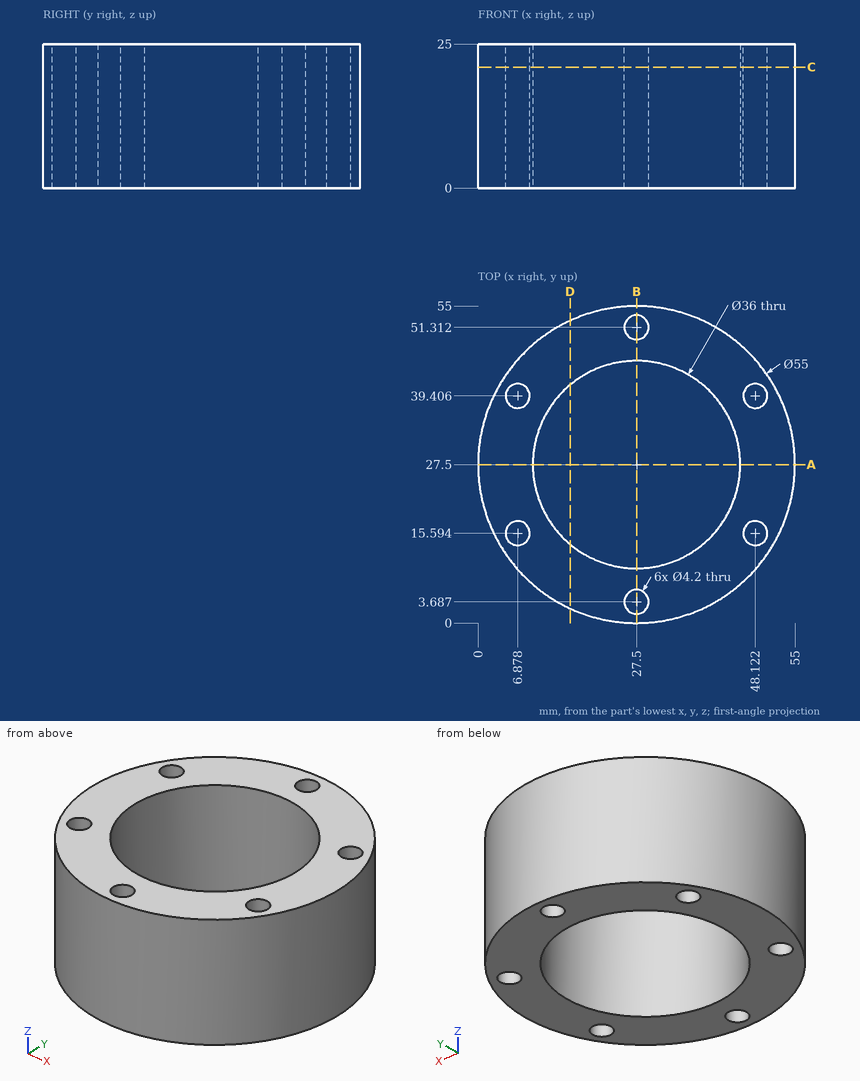
Geometry check sheet. Reference: drawing and pictorial views, mm from the part's lowest x, y, z. Give positions to 0.01 mm unless a question says otherwise; leave off trailing zeros. Write each loop counter-clockwise with the first axis right and the second up, starting at its lowest first coordinate (ties: lowest second). Pieces come first, ordered by that corner, then holes.
Item 1: Gauge pin test, flat ends, axial feed: pin 1 (4 mm diameter, centred on x = 48.12, y = 15.59, fed in from +Z); pin 2 (4 mm diameter, centred on x = 24, z = 15, fed in from -Y); pin 3 (8 mm diameter, centred on x = 6, y = 38, fed in from +Z); pin 4 (1.5 mm diameter, centred on x = 22.5, z = 14.5, fed in from +Y). Record the tip position at first contact, or that the pin passes through.
Item 2: Cross-section at A-A (y = 27.5). Enter the section's corners in (x, z), and give its area (3 significant figures).
Item 3: Cross-section at C-C (z = 21). Enter the section's corners in (x, y) (1 decimal).
Item 4: Cross-section at B-B (x = 27.5). Enter the section's corners in (y, z), and give its area (3 significant figures).
Item 5: Cross-section at D-D (x = 16). Enter the section's corners in (y, z).
Item 6: Scan lines: L1, parallel to Y at x = 27.5, z = 11; L2, parallel to X at y = 17.5, z = 8 (1 decimal); L3, parallel to Y at x = 27, z = 9 (1 decimal). Record each from-to range of solid material in increasing order.
Report:
1. pin 1: passes through
1. pin 2: stops at y = 0.04
1. pin 3: stops at z = 25
1. pin 4: stops at y = 54.67
2. outline: (0, 0) - (9.5, 0) - (9.5, 25) - (0, 25) - close; (45.5, 0) - (55, 0) - (55, 25) - (45.5, 25) - close
2. area: 475 mm2
3. outline: circle Ø55 at (27.5, 27.5); hole circle Ø4.2 at (6.9, 15.6); hole circle Ø4.2 at (6.9, 39.4); hole circle Ø36 at (27.5, 27.5); hole circle Ø4.2 at (27.5, 3.7); hole circle Ø4.2 at (27.5, 51.3); hole circle Ø4.2 at (48.1, 15.6); hole circle Ø4.2 at (48.1, 39.4)
4. outline: (0, 0) - (1.59, 0) - (1.59, 25) - (0, 25) - close; (5.79, 0) - (9.5, 0) - (9.5, 25) - (5.79, 25) - close; (45.5, 0) - (49.21, 0) - (49.21, 25) - (45.5, 25) - close; (53.41, 0) - (55, 0) - (55, 25) - (53.41, 25) - close
4. area: 265 mm2
5. outline: (2.52, 0) - (13.65, 0) - (13.65, 25) - (2.52, 25) - close; (41.35, 0) - (52.48, 0) - (52.48, 25) - (41.35, 25) - close
6. L1: y = 0 to 1.59, 5.79 to 9.5, 45.5 to 49.21, 53.41 to 55
6. L2: x = 1.9 to 6, 7.8 to 12.5, 42.5 to 47.2, 49 to 53.1
6. L3: y = 0 to 1.6, 5.7 to 9.5, 45.5 to 49.3, 53.4 to 55
